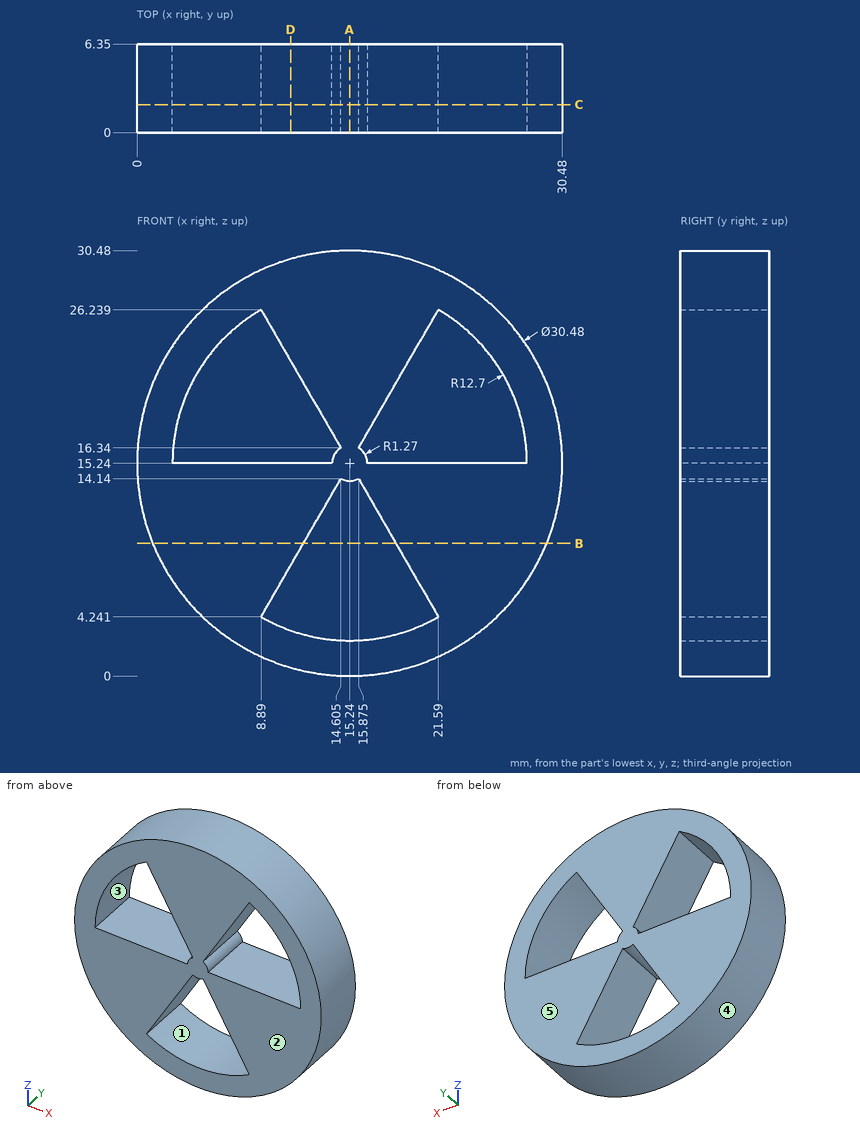
Here's the drawing with two shaded views (mm, measured from the low corner). I have some questions. A direction names the side the tool comes from. Round coordinates to 2 decimals unless told otherwise and drop trailing zeros. Loops run counter-clockwise (first coordinate to the right, second up) from the corner with the lowest first, then second, coordinate; pieces in that order, holes last.
Item 1: Suppose I cut it at B-B, the plane z = 9.5. Write out the boundary of the cut face in (x, y), then the cut area to 3 significant figures.
Item 2: If we mould it in two halves opening along Z, with no side actions, what happens to the marked faces 3, 4 and 5? For each: +Z half, -Z half, draft (parallel to the pull), parting line (faces both ways), or undercut.
Item 3: Will these pins go through, and if not, where does the flat tip stop? pin 1 Ø3 at (y, z) = (2.5, 17.5) entering from +X; pin 2 Ø1.9 at (x, y) = (10, 1.5) entering from +Z; pin 3 Ø1 at (x, y) = (11, 1.5) entering from +Z.
Item 4: Suppose I cut it at C-C, the plane y = 2. Write out the boundary of the cut face in (x, z) (1 decimal), then the cut area to 3 significant figures.
Item 5: Which directions (+Z, -Z, +X, -X, +Y, -Y) give clear straight access to the entire face, cutting with the end or side of a thin tool? Please do the marked faces 1 and 2.
Item 6: Suppose I cut it at D-D, the plane x = 11. Write out the boundary of the cut face in (y, z).
Item 7: Please list where these lines run through material, in increasing order: L1, parallel to Z at x = 14.5, y = 5.5 (1 decimal); L2, parallel to X at y = 2, z = 25.5 (1 decimal); L3, parallel to X at y = 3, z = 20 (1 decimal).
Item 8: Suppose I cut it at A-A, the plane x = 15.24. Write out the boundary of the cut face in (y, z), then the cut area to 3 significant figures.
Reported:
1. outline: (1.12, 0) - (11.93, 0) - (11.93, 6.35) - (1.12, 6.35) - close; (18.55, 0) - (29.36, 0) - (29.36, 6.35) - (18.55, 6.35) - close
1. area: 137 mm2
2. face 3: undercut
2. face 4: parting line
2. face 5: draft
3. pin 1: stops at x = 30.46
3. pin 2: stops at z = 29.86
3. pin 3: stops at z = 30.01
4. outline: circle Ø30.5 at (15.2, 15.2); hole (2.5, 15.2) - (14, 15.2) arc R1.3 cw to (14.6, 16.3) - (8.9, 26.2) arc R12.7 ccw to start; hole (8.9, 4.2) arc R12.7 ccw to (21.6, 4.2) - (15.9, 14.1) arc R1.3 cw to (14.6, 14.1) - close; hole (15.9, 16.3) arc R1.3 cw to (16.5, 15.2) - (27.9, 15.2) arc R12.7 ccw to (21.6, 26.2) - close
4. area: 479 mm2
5. face 1: +Y, -Y
5. face 2: +Z, -Z, +X, -X, -Y
6. outline: (0, 0.6) - (6.35, 0.6) - (6.35, 3.27) - (0, 3.27) - close; (0, 7.9) - (6.35, 7.9) - (6.35, 15.24) - (0, 15.24) - close; (0, 22.58) - (6.35, 22.58) - (6.35, 29.88) - (0, 29.88) - close
7. L1: z = 0 to 2.6, 14 to 16.3, 16.5 to 30.5
7. L2: x = 4 to 7.8, 9.3 to 21.2, 22.7 to 26.5
7. L3: x = 0.8 to 3.5, 12.5 to 18, 27 to 29.7
8. outline: (0, 0) - (6.35, 0) - (6.35, 2.54) - (0, 2.54) - close; (0, 13.97) - (6.35, 13.97) - (6.35, 30.48) - (0, 30.48) - close
8. area: 121 mm2
